Autodesk Fusion 360 part; units mm, degrees
sketch "Sketch1" plane through (0, 0, 0) normal (0, 0, 1) x (1, 0, 0)
  line L0 (65, 55) -> (-65, 55)
  line L1 (-65, 55) -> (-65, -55)
  line L2 (-65, -55) -> (65, -55)
  line L3 (65, -55) -> (65, 55)
  line L4 (65, 55) -> (-65, -55) construction
  line L5 (-65, 55) -> (65, -55) construction
  line L6 (61.5, 51.5) -> (-61.5, 51.5)
  line L7 (-61.5, 51.5) -> (-61.5, -51.5)
  line L8 (-61.5, -51.5) -> (61.5, -51.5)
  line L9 (61.5, -51.5) -> (61.5, 51.5)
  line L10 (61.5, 51.5) -> (-61.5, -51.5) construction
  line L11 (-61.5, 51.5) -> (61.5, -51.5) construction
  circle A0 centre (-61.5, 51.5) radius 3.5
  circle A1 centre (61.5, 51.5) radius 3.5
  circle A2 centre (61.5, -51.5) radius 3.5
  circle A3 centre (-61.5, -51.5) radius 3.5
  circle A4 centre (-61.5, -51.5) radius 1.75
  circle A5 centre (61.5, -51.5) radius 1.75
  circle A6 centre (61.5, 51.5) radius 1.75
  circle A7 centre (-61.5, 51.5) radius 1.75
  circle A8 centre (0, 0) radius 38.5
  line L12 (30.25, 30.25) -> (-30.25, 30.25)
  line L13 (-30.25, 30.25) -> (-30.25, -30.25)
  line L14 (-30.25, -30.25) -> (30.25, -30.25)
  line L15 (30.25, -30.25) -> (30.25, 30.25)
  line L16 (30.25, 30.25) -> (-30.25, -30.25) construction
  line L17 (-30.25, 30.25) -> (30.25, -30.25) construction
  circle A9 centre (30.25, 30.25) radius 2
  circle A10 centre (-30.25, 30.25) radius 2
  circle A11 centre (-30.25, -30.25) radius 2
  circle A12 centre (30.25, -30.25) radius 2
  dimension "d1" = 130
  dimension "d2" = 110
  dimension "d3" = 3.5
  dimension "d4" = 3.5
  dimension "d5" = 3.5
  dimension "d6" = 3.5
  dimension "d7" = 3.5
  dimension "d8" = 3.5
  dimension "d9" = 77
  dimension "d10" = 60.5
  dimension "d11" = 60.5
  dimension "d12" = 4
  dimension "d13" = 4
  dimension "d14" = 4
  dimension "d15" = 4
extrude "Extrude1" add sketch "Sketch1" along normal blind 3 contours L0 L6 A0 A1 | L6 L9 A1 A6 | L3 L9 A1 A2 | L6 L7 A0 A7 | L6 L7 L8 L9 A0 A1 A2 A3 | L6 L9 A1 A6 | L8 L9 A2 A5 | L6 L7 A0 A7 | L1 L7 A0 A3 | L8 L9 A2 A5 | L2 L8 A2 A3 | L7 L8 A3 A4 | L7 L8 A3 A4 | A8 L12 L15 A9 | A8 L14 L15 A12 | A8 L12 L13 A10 | A8 L13 L14 A11
Could you check a few things on this model? Use its own coordinates, in mm. Coordinates: 2 decimals unless noted, no trailing zeros. Write each loop counter-clockwise with the first axis right and the second up, starting at its lowest first coordinate (ties: lowest second). Pieces come first, ordered by that corner, then holes. Notation, with made-up numbers: (-29.5, -26) - (0.5, -26) arc R34 cw to (0.5, 9) - close; hole circle Ø11 at (-20.75, 77). An arc over 180 degrees is marked (long way). Write item = value, one per line.
1) Please list where these lines run through material, in increasing order: line 1 (Y direction, x = 61.5, z = 1.4); line 2 (X direction, y = 51.5, z = 1.2); line 3 (X direction, y = 0, z = 2.1). Write a range as [from, to].
Result set:
line_1 = [-55, -53.25], [-49.75, 49.75], [53.25, 55]
line_2 = [-65, -63.25], [-59.75, 59.75], [63.25, 65]
line_3 = [-65, -38.5], [38.5, 65]
2) Suppose I cut it at A-A on x = 0. Please give me the cut outline in (y, z), plus the area to 3 significant figures.
Result set:
outline = (-55, 0) - (-38.5, 0) - (-38.5, 3) - (-55, 3) - close; (38.5, 0) - (55, 0) - (55, 3) - (38.5, 3) - close
area = 99.0 mm2
3) Suppose I cut it at B-B on y = 14. Please give me the cut outline in (x, z), plus the area to 3 significant figures.
Result set:
outline = (-65, 0) - (-35.86, 0) - (-35.86, 3) - (-65, 3) - close; (35.86, 0) - (65, 0) - (65, 3) - (35.86, 3) - close
area = 175 mm2
4) Suppose I cut it at C-C on z = 2.5. State how many separate pieces and enclosed holes the cut face has, plus the area to 3 significant figures.
Result set:
separate_pieces = 1
enclosed_holes = 9
area = 9,540 mm2
5) We'd pull the mould along X, two halves only. Please class faces 1 (the cylindrical face through (-64, 53.95, 1.48)), 2 (the cylindrical face through (63.117, -50.83, 1.479)), 3 (the flat face through (-30, 25, 3)): +X half, -X half, draft (parallel to the pull), parting line (faces both ways), or undercut.
Result set:
face_1 = -X half
face_2 = undercut
face_3 = draft
6) Suppose I cut it at D-D on x = -30.25. Please give me the cut outline in (y, z), plus the area to 3 significant figures.
Result set:
outline = (-55, 0) - (-32.25, 0) - (-32.25, 3) - (-55, 3) - close; (-28.25, 0) - (-23.82, 0) - (-23.82, 3) - (-28.25, 3) - close; (23.82, 0) - (28.25, 0) - (28.25, 3) - (23.82, 3) - close; (32.25, 0) - (55, 0) - (55, 3) - (32.25, 3) - close
area = 163 mm2
